from build123d import *

# Parameters (mm, degrees)
BOSS_EXTRUDE4_DEPTH    = 13.716
CUT_EXTRUDE2_START     = 13.394831099
CUT_EXTRUDE2_OUTLINE_W = 71
CUT_EXTRUDE2_OUTLINE_H = 102
CUT_EXTRUDE2_DEPTH     = 19.052275388
BOSS_EXTRUDE7_DEPTH    = 12.7


# Read off the part's stored shape, not the designer's step: Cut-Extrude2
with BuildPart() as part:
    # Sketch2 → Boss-Extrude4 (new body)
    with BuildSketch(Plane(origin=(0, 0, 0), x_dir=(1, 0, 0), z_dir=(0, 1, 0))):
        with BuildLine():
            Line((0, 0), (13.212422732, 31.078396728))
            ThreePointArc((13.212422732, 31.078396728), (47.046788058, 4.181077282), (67.884833627, -33.687193436))
            Line((67.884833627, -33.687193436), (67.884833627, -66.675))
            Line((67.884833627, -66.675), (39.309833627, -66.675))
            ThreePointArc((39.309833627, -66.675), (28.750791411, -27.974810579), (0, 0))
        make_face()
    extrude(amount=BOSS_EXTRUDE4_DEPTH)

    # Cut-Extrude2 outline → Cut-Extrude2 (cut)
    with BuildSketch(Plane(origin=(0, 0, 0), x_dir=(0.9802048878944475, -0.19725451306837943, -0.017001024145327306), z_dir=(0.19798580188446208, 0.9765843612447384, 0.08417011122942132)).offset(CUT_EXTRUDE2_START)):
        with Locations((31.5, -17)):
            Rectangle(CUT_EXTRUDE2_OUTLINE_W, CUT_EXTRUDE2_OUTLINE_H)
    extrude(amount=CUT_EXTRUDE2_DEPTH, mode=Mode.SUBTRACT)

    # Sketch16 → Boss-Extrude7 (add)
    with BuildSketch(Plane.XZ):
        with BuildLine():
            Line((32.238416067, 34.617565762), (48.16212184, -2.83833884))
            ThreePointArc((48.16212184, -2.83833884), (60.654452135, -7.877479025), (65.69359232, 4.614851269))
            Line((65.69359232, 4.614851269), (60.724626835, 16.302903023))
            Line((60.724626835, 16.302903023), (39.309833627, 66.675))
            ThreePointArc((39.309833627, 66.675), (26.817503332, 71.714140186), (21.778363147, 59.221809891))
            Line((21.778363147, 59.221809891), (32.238416067, 34.617565762))
        make_face()
        with BuildLine():
            Line((10.740738204, 7.196121991), (24.250560746, -24.581821632))
            Line((24.250560746, -24.581821632), (24.900069719, -26.109603322))
            ThreePointArc((24.900069719, -26.109603322), (21.540642929, -34.437823519), (13.212422732, -31.078396728))
            Line((13.212422732, -31.078396728), (0, 0))
            Line((0, 0), (-0.946908783, 2.227328585))
            ThreePointArc((-0.946908783, 2.227328585), (2.412518007, 10.555548781), (10.740738204, 7.196121991))
        make_face()
    extrude(amount=BOSS_EXTRUDE7_DEPTH)


solid = part.part
Input: part model. Units: mm. Frame: model coordinates. A direction names the side the tool comes from. Round coordinates to 2 decimals unless told otherwise and drop trailing zeros. Order: outer loops, then holes, each group sorted by start corner. A loop starts at its lowest first (then second) coordinate and runs counter-clockwise, first axis right, second up.
1. Cut plane B-B, the plane x = 17. Output: boundary loops of the cut face in (y, z), then the cut area to 3 significant figures.
The answers:
outline: (-12.7, -34.6) - (0, -34.6) - (0, -29.04) - (12.77, -29.04) - (9.17, 12.8) - (0, 12.8) - (0, -7.53) - (-12.7, -7.53) - close
area: 803 mm2
2. Pin query (flat end, axial travel): P1, Ø11, axis at x = 22.5, z = 2, coming from the -Y side; P2, Ø3, axis at x = 58.5, z = 10.5, coming from the +Y side; P3, Ø3.5, axis at x = 6, z = 4.5, coming from the +Y side. Return the tip coordinate at first contact, or that it passes through.
The answers:
P1: stops at y = 0
P2: stops at y = 1.28
P3: stops at y = 12.43
3. Cut plane C-C, the plane z = 27.5. Output: boundary loops of the cut face in (x, y).
The answers:
outline: (28.47, 0) - (35.26, 0) - (35.26, -12.7) - (55.96, -12.7) - (55.96, 0) - (28.47, 5.57) - close
4. Cut plane D-D, the plane x = 38. Output: boundary loops of the cut face in (y, z).
The answers:
outline: (-12.7, 21.07) - (0, 21.07) - (0, -13.68) - (7.19, -13.68) - (1.48, 52.61) - (0, 52.61) - (0, 68.88) - (-12.7, 68.88) - close
5. Cut plane A-A, the plane y = -3.25. Output: boundary loops of the cut face in (x, z) (3 decimals), then the cut area to 3 significant figures.
The answers:
outline: (-0.947, 2.227) - (13.212, -31.078) arc R6.35 ccw to (24.9, -26.11) - (10.741, 7.196) arc R6.35 ccw to start; (21.778, 59.222) - (48.162, -2.838) arc R9.525 ccw to (65.694, 4.615) - (39.31, 66.675) arc R9.525 ccw to start
area: 2,160 mm2
6. Mould query, pull axis X, two halves, no side actions, for faces 1 (the face through (28.86, 5.24, -21.32)), 2 (the face through (30, 0, 5)), 3 (the face through (12, -12.7, -12)). Classes: released by +X, released by -X, zero draft, split by the parting line, or undercut.
The answers:
face 1: released by +X
face 2: undercut
face 3: zero draft
7. Set-up query: faces 4 (the face through (59, 0, 1)), 5 (the face through (29.937, 7.118, 6.135)), 6 (the face through (3, 0, 7)). Return all of +Z, -Z, +X, -X, +Y, -Y with unobstructed straight access to the full face (end or side cutting, diameter ignored); none if empty.
The answers:
face 4: -Z, +X, +Y
face 5: +Z, +X, +Y
face 6: +Z, -X, +Y
8. Material intervals for line 1 (Y direction, x = 62, z = -7); line 2 (X direction, y = -5.75, z = -17.5); line 3 (X direction, y = -8, z = -6), sorted ascending.
The answers:
line 1: y = -12.7 to 0
line 2: x = 7.44 to 21.24
line 3: x = 2.55 to 16.35, 50.35 to 63.51
